Can you work these out from the model? Positions are in its coordinate system, mm. Face numbers are marked on the shaded views. A direction names the side the tool comes from. Give positions to 0.01 mm unless a question says otherwise; leave off trailing zeros. Write each loop counter-clockwise with the first axis right and the second up, starting at its lowest first coordinate (ties: lowest second). Pieces come first, ordered by that corner, then holes. Notation, with made-up numbers: (49.25, 19) - (82.25, 19) arc R9 cw to (82.25, 26) - close; hole circle Ø7 at (43, 43.5). An arc over 180 degrees is marked (long way). Use a Markdown table: item, result. Add a question column.
```python
from build123d import *

# Parameters (mm, degrees)
BOSS_EXTRUDE1_DEPTH = 19.5
CUT_EXTRUDE2_DEPTH  = 14.5
CUT_EXTRUDE3_DEPTH  = 42.05179655
CUT_EXTRUDE4_DEPTH  = 42.05179655


with BuildPart() as part:
    # Sketch1 → Boss-Extrude1 (new body)
    with BuildSketch(Plane.XY):
        Polygon((0, 0), (0, 27), (5, 27), (5, 22.5), (22.5, 5), (27, 5), (27, 0), align=None)
    extrude(amount=BOSS_EXTRUDE1_DEPTH)

    # Sketch2 → Cut-Extrude2 (cut)
    with BuildSketch(Plane.XY.offset(17)):
        Polygon((3, 27), (5, 27), (5, 22.5), (22.5, 5), (27, 5), (27, 3), (3, 3), align=None)
    extrude(amount=-CUT_EXTRUDE2_DEPTH, mode=Mode.SUBTRACT)

    # Sketch3 → Cut-Extrude3 (cut, through all)
    with BuildSketch(Plane(origin=(0, 3, 0), x_dir=(1, 0, 0), z_dir=(0, 1, 0))):
        with BuildLine():
            Line((13, -6.25), (17, -6.25))
            ThreePointArc((17, -6.25), (20.5, -9.75), (17, -13.25))
            Line((17, -13.25), (13, -13.25))
            ThreePointArc((13, -13.25), (9.5, -9.75), (13, -6.25))
        make_face()
    extrude(amount=-CUT_EXTRUDE3_DEPTH, mode=Mode.SUBTRACT)

    # Sketch4 → Cut-Extrude4 (cut, through all)
    with BuildSketch(Plane(origin=(3, 0, 0), x_dir=(0, 0, -1), z_dir=(1, 0, 0))):
        with BuildLine():
            Line((-13.25, 13), (-13.25, 17))
            ThreePointArc((-13.25, 17), (-9.75, 20.5), (-6.25, 17))
            Line((-6.25, 17), (-6.25, 13))
            ThreePointArc((-6.25, 13), (-9.75, 9.5), (-13.25, 13))
        make_face()
    extrude(amount=-CUT_EXTRUDE4_DEPTH, mode=Mode.SUBTRACT)


solid = part.part
```
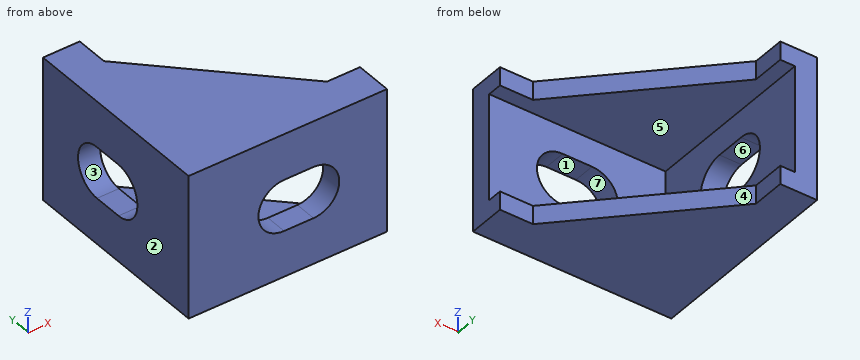
Q1. Suppose I cut it at A-A (x = 15). Please give me the cut outline in (y, z).
Q2. I'm going to push flat-ended pins straight in: P1, Ø5, axis at x = 14.5, z = 7, coming from the +Y side; P2, Ø0.8, axis at x = 25, z = 18, coming from the +Y side; P3, Ø0.8, axis at y = 24, z = 18.5, coming from the +X side. Where does each tip first touch, or does it pass through?
Q3. If I drill on probe 1 along Z at (x, y) = (17.5, 5.5); probe 2 along Y at (x, z) = (17.25, 5); probe 3 along Y at (x, z) = (10.5, 18.5), over which ranges is the centre line in solid material (lowest first)? Write a range as [from, to].
Q4. Suppose I cut it at C-C (x = 6.5). Please give me the cut outline in (y, z), and give its area (4 significant figures).
Q5. Suppose I cut it at D-D (y = 17.75). Please give me the cut outline in (x, z).
Q6. Suppose I cut it at B-B (z = 9.75). Please give me the cut outline in (x, y), and give its area (3 significant figures).
Q7. On a 3-axis mill with a long thin cutter (end or side, diameter ignored), from which of +Z, -Z, +X, -X, +Y, -Y can I reach the whole of each face in a straight line? I mean the marked faces 5, 6 and 7. Say none if no direction works.
Q8. If we mould it in two halves opening along X, with no side actions, what happens to the marked faces 1, 2, 3 and 4? For each: released by +X, released by -X, zero draft, split by the parting line, or undercut.
Derived:
| question | item | result |
|---|---|---|
| 1 | outline | (0, 0) - (12.5, 0) - (12.5, 2.5) - (3, 2.5) - (3, 6.25) - (0, 6.25) - close; (0, 13.25) - (3, 13.25) - (3, 17) - (12.5, 17) - (12.5, 19.5) - (0, 19.5) - close |
| 2 | P1 | y = 3 |
| 2 | P2 | y = 5 |
| 2 | P3 | x = 5 |
| 3 | probe 1 | [0, 2.5], [17, 19.5] |
| 3 | probe 2 | [0, 3] |
| 3 | probe 3 | [0, 17] |
| 4 | outline | (0, 0) - (21, 0) - (21, 2.5) - (3, 2.5) - (3, 17) - (21, 17) - (21, 19.5) - (0, 19.5) - close |
| 4 | area | 148.5 mm² |
| 5 | outline | (0, 0) - (9.75, 0) - (9.75, 2.5) - (3, 2.5) - (3, 6.33) - (0, 6.33) - close; (0, 13.17) - (3, 13.17) - (3, 17) - (9.75, 17) - (9.75, 19.5) - (0, 19.5) - close |
| 6 | outline | (0, 0) - (9.5, 0) - (9.5, 3) - (3, 3) - (3, 9.5) - (0, 9.5) - close; (0, 20.5) - (3, 20.5) - (3, 27) - (0, 27) - close; (20.5, 0) - (27, 0) - (27, 3) - (20.5, 3) - close |
| 6 | area | 87.0 mm² |
| 7 | face 5 | +X, +Y |
| 7 | face 6 | +X, -X |
| 7 | face 7 | +Y, -Y |
| 8 | face 1 | undercut |
| 8 | face 2 | released by -X |
| 8 | face 3 | zero draft |
| 8 | face 4 | released by +X |
